The drawing under review shows one solid part. Ordinate dimensions are in mm from its lowest x, y, z. A direction names the side the tool comes from. Coordinates: 2 decimals unless noted, no trailing zeros. Loops run counter-clockwise (first coordinate to the right, second up) from the corner with the lowest first, then second, coordinate; pieces in that order, holes last. Notation, with made-up numbers: M 5.25,-13 L 29.25,-13 A7 cw 29.25,-7 Z; hole C 70,22.5 d3. An arc over 180 degrees is marked long. Put each result on its own line as item: value.
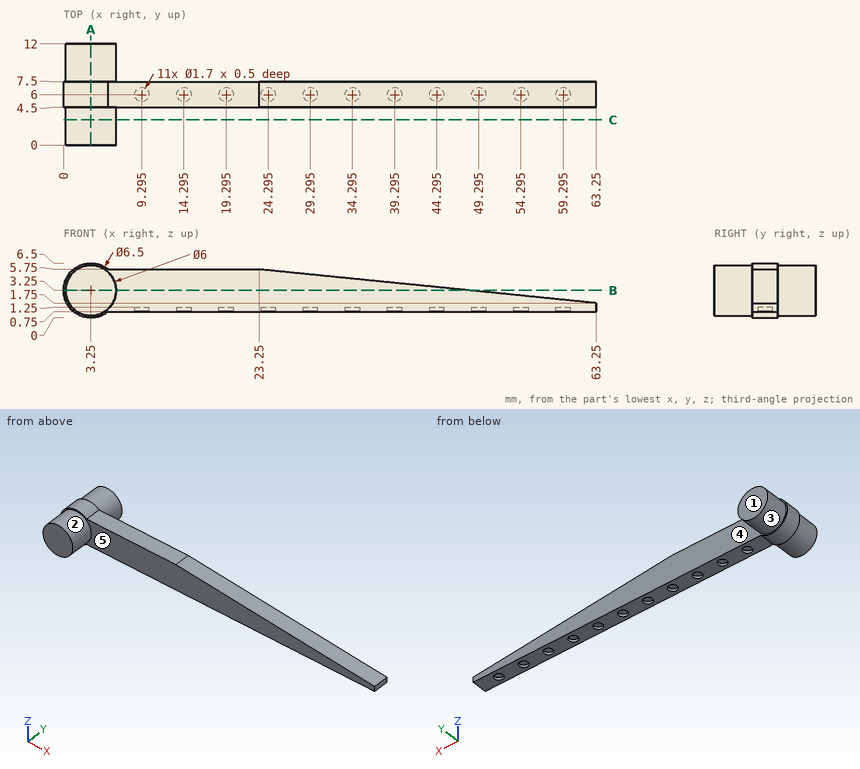
(1) For pin 1 (2 mm diameter, centred on x = 14.29, y = 6, fed in from -Z); pin 2 (0.5 mm diameter, centred on x = 29.5, y = 6, fed in from -Z); pin 3 (2 mm diameter, centred on x = 40.5, z = 4, fed in from +Y), all flat-tipped, find the tip position at first contact; note any pin that passes through.
Determined:
pin 1: stops at z = 0.75
pin 2: stops at z = 1.25
pin 3: stops at y = 7.5
(2) Draft analysis for pull direction Y (two halves, no side actions). For the marked faces 3, 4 and 5, state which applies: +Y half, -Y half, draft (parallel to the pull), parting line (faces both ways), or undercut.
Determined:
face 3: draft
face 4: +Y half
face 5: -Y half
(3) Add section B-B (z = 3.25). Write out the cut boundary in (x, y), plus the area to 3 significant figures.
Determined:
outline: M 0,4.5 L 0.25,4.5 L 0.25,0 L 6.25,0 L 6.25,4.5 L 48.25,4.5 L 48.25,7.5 L 6.25,7.5 L 6.25,12 L 0.25,12 L 0.25,7.5 L 0,7.5 Z
area: 199 mm^2
(4) Add section A-A (x = 3.25). Write out the cut boundary in (y, z).
Determined:
outline: M 0,0.25 L 4.5,0.25 L 4.5,0 L 7.5,0 L 7.5,0.25 L 12,0.25 L 12,6.25 L 7.5,6.25 L 7.5,6.5 L 4.5,6.5 L 4.5,6.25 L 0,6.25 Z
(5) Tool access review of the marked faces 1 and 2: name each direction out of +Z, -Z, +X, -X, +Y, -Y from which nothing blocks a thin tool from reaching the whole face with its end or side.
Determined:
face 1: +Z, -Z, +X, -X, +Y
face 2: -Y
(6) Wall thickness on line 1 along Y through (x, z) = (30, 1.75); line 2 along X through (y, z) = (2, 1.5); line 3 along X through (y, z) = (7.75, 6): over which ranges is each line inside the solid? List them lowest first. Write a range as [from, to].
Determined:
line 1: y = [4.5, 7.5]
line 2: x = [0.81, 5.69]
line 3: x = [2.05, 4.45]
(7) Add section C-C (y = 3). Write out the cut boundary in (x, z), plus the area to 3 significant figures.
Determined:
outline: C 3.25,3.25 d6
area: 28.3 mm^2
